from build123d import *

# Parameters (mm, degrees)
SKETCH_W      = 52
SKETCH_H      = 52
SKETCH_R      = 1.8
SKETCH_R_2    = 1.2
SKETCH_W_2    = 38
SKETCH_H_2    = 11.5
PAD_DEPTH     = 2
SKETCH001_R   = 2
SKETCH001_R_2 = 2.75
SKETCH001_R_3 = 1.2
PAD001_DEPTH  = 4.5
SKETCH002_W   = 17
SKETCH002_H   = 16
POCKET_DEPTH  = 5


with BuildPart() as part:
    # Sketch → Pad (new body)
    with BuildSketch(Plane.XY):
        Rectangle(SKETCH_W, SKETCH_H)
        with Locations((22.25, 22.25)):
            Circle(SKETCH_R, mode=Mode.SUBTRACT)
        with Locations((22.25, -22.25)):
            Circle(SKETCH_R, mode=Mode.SUBTRACT)
        with Locations((-22.25, 22.25)):
            Circle(SKETCH_R, mode=Mode.SUBTRACT)
        with Locations((-22.25, -22.25)):
            Circle(SKETCH_R, mode=Mode.SUBTRACT)
        with Locations((-10.35, 15.5)):
            Circle(SKETCH_R_2, mode=Mode.SUBTRACT)
        with Locations((10.35, 15.5)):
            Circle(SKETCH_R_2, mode=Mode.SUBTRACT)
        with Locations((0, -13.25)):
            Rectangle(SKETCH_W_2, SKETCH_H_2, mode=Mode.SUBTRACT)
    extrude(amount=PAD_DEPTH)

    # Sketch001 → Pad001 (new body)
    with BuildSketch(Plane.XY.offset(2)):
        with Locations((0, -5.4)):
            Circle(SKETCH001_R)
        with Locations((-10.35, 15.5)):
            Circle(SKETCH001_R_2)
        with Locations((-10.35, 15.5)):
            Circle(SKETCH001_R_3, mode=Mode.SUBTRACT)
        with Locations((10.35, 15.5)):
            Circle(SKETCH001_R_2)
        with Locations((10.35, 15.5)):
            Circle(SKETCH001_R_3, mode=Mode.SUBTRACT)
    extrude(amount=PAD001_DEPTH)

    # Sketch002 → Pocket (cut)
    with BuildSketch(Plane.XY.offset(2)):
        with Locations((-10.5, 3.5)):
            Rectangle(SKETCH002_W, SKETCH002_H)
        with Locations((10.5, 3.5)):
            Rectangle(SKETCH002_W, SKETCH002_H)
    extrude(amount=-POCKET_DEPTH, mode=Mode.SUBTRACT)


solid = part.part
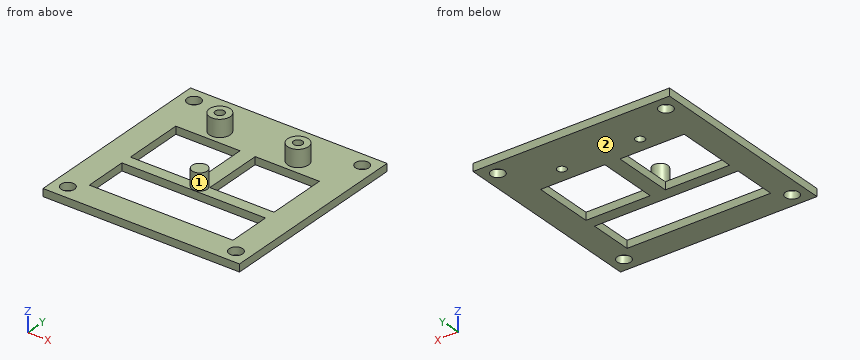
CAD build for the part. Positions are in the model's coordinates, mm. Face numbers are marked on the shaded views. A direction names the side the tool comes from. Round coordinates to 2 decimals unless told otherwise and drop trailing zeros. Order: outer loops, then holes, each group sorted by start corner. A loop starts at its lowest first (then second) coordinate and runs counter-clockwise, first axis right, second up. Notation, with made-up numbers: M -33,13 L -17,13 A32 ccw -17,44 Z; hole C 59,22.25 d6. An arc over 180 degrees is marked long. Use one line per item in the form item = value.
Q1. Flat gauge pins, fed straight in: P1, Ø1, axis at y = -12, z = 3.5, coming from the -X side; P2, Ø6, axis at x = -22.25, y = -22.25, coming from the +Z side; P3, Ø3, axis at x = -12.5, z = 4, coming from the -Y side. Where does each tip first touch, or does it go through?
Recorded:
P1 = through
P2 = 2
P3 = 12.83
Q2. Saw through at D-D on x = -22.25. Give the cut face in (y, z), then the cut area to 3 significant figures.
Recorded:
outline = M -26,0 L -24.05,0 L -24.05,2 L -26,2 Z; M -20.45,0 L 20.45,0 L 20.45,2 L -20.45,2 Z; M 24.05,0 L 26,0 L 26,2 L 24.05,2 Z
area = 89.6 mm^2
Q3. Saw through at B-B on z = 5.75. Give the cut face in (x, y), then the cut area to 3 significant figures.
Recorded:
outline = C -10.35,15.5 d5.5; C 0,-5.4 d4; C 10.35,15.5 d5.5; hole C -10.35,15.5 d2.4; hole C 10.35,15.5 d2.4
area = 51.0 mm^2
Q4. Saw through at A-A on x = 10.35. Give the cut face in (y, z), then the cut area to 4 significant figures.
Recorded:
outline = M -26,0 L -19,0 L -19,2 L -26,2 Z; M -7.5,0 L -4.5,0 L -4.5,2 L -7.5,2 Z; M 11.5,0 L 14.3,0 L 14.3,6.5 L 12.75,6.5 L 12.75,2 L 11.5,2 Z; M 16.7,0 L 26,0 L 26,2 L 18.25,2 L 18.25,6.5 L 16.7,6.5 Z
area = 58.15 mm^2
Q5. Saw through at C-C on y = 15.5. Give the cut face in (x, z), then the cut area to 3 significant figures.
Recorded:
outline = M -26,0 L -11.55,0 L -11.55,6.5 L -13.1,6.5 L -13.1,2 L -26,2 Z; M -9.15,0 L 9.15,0 L 9.15,6.5 L 7.6,6.5 L 7.6,2 L -7.6,2 L -7.6,6.5 L -9.15,6.5 Z; M 11.55,0 L 26,0 L 26,2 L 13.1,2 L 13.1,6.5 L 11.55,6.5 Z
area = 122 mm^2
Q6. Probe L1, parallel to X at y = 6.5, z = 0.75; L2, parallel to Y at x = 22.25, z = 1.1; L3, parallel to Y at x = 14, z = 1.5. List the from-to ranges inside material, lowest first.
Recorded:
L1 = -26 to -19, -2 to 2, 19 to 26
L2 = -26 to -24.05, -20.45 to 20.45, 24.05 to 26
L3 = -26 to -19, -7.5 to -4.5, 11.5 to 26
Q7. Which spindle directions (+Z, -Z, +X, -X, +Y, -Y) get a long thin tool onto all of the face, cutting with end or side? Do the marked faces 1 and 2. Say none if no direction does.
Recorded:
face_1 = +Z
face_2 = -Z, +X, -X, +Y, -Y
